Can you work these out from the model? Positions are in its coordinate system, mm. A direction names the side the tool comes from. Give positions to 0.01 mm unless a question says otherwise; leave off trailing zeros. Loops run counter-clockwise (first coordinate to the right, second up) from the corner with the lowest first, then second, coordinate; pieces in that order, holes last. Notation, with made-up numbers: (14.5, -32.75) -> (57.5, -32.75) arc R19 cw to (57.5, -22.75) -> close; hole circle Ø4 at (72, 81.5). An arc over 180 degrees is marked (long way). Use CSV: the item, a comma, the result in double quotes.
from build123d import *

# Parameters (mm, degrees)
SKIZZE1_W                            = 100
SKIZZE1_H                            = 25
AUFSATZ_LINEAR_AUSTRAGEN1_DEPTH      = 3
SKIZZE3_W                            = 4
SKIZZE3_H                            = 17
AUFSATZ_LINEAR_AUSTRAGEN2_DEPTH      = 17
SCHNITT_LINEAR_AUSTRAGEN1_DEPTH      = 78.95222289
SCHNITT_LINEAR_AUSTRAGEN1_DEPTH_BACK = 78.95222289
SKIZZE5_R                            = 2.55
VERRUNDUNG1_R                        = 8.5
SKIZZE6_R                            = 2.6
SCHNITT_LINEAR_AUSTRAGEN2_DEPTH      = 3
VERRUNDUNG2_R                        = 1


with BuildPart() as part:
    # Skizze1 → Aufsatz-Linear austragen1 (new body)
    with BuildSketch(Plane.XY):
        with Locations((45.947748482, 6.142667555)):
            Rectangle(SKIZZE1_W, SKIZZE1_H)
    extrude(amount=AUFSATZ_LINEAR_AUSTRAGEN1_DEPTH)

    # Skizze3 → Aufsatz-Linear austragen2 (add)
    with BuildSketch(Plane.XY.offset(3)):
        with Locations((12.947748482, 6.142667555)):
            Rectangle(SKIZZE3_W, SKIZZE3_H)
        with Locations((20.947748482, 6.142667555)):
            Rectangle(SKIZZE3_W, SKIZZE3_H)
        with Locations((78.947748482, 6.142667555)):
            Rectangle(SKIZZE3_W, SKIZZE3_H)
        with Locations((70.947748482, 6.142667555)):
            Rectangle(SKIZZE3_W, SKIZZE3_H)
    extrude(amount=AUFSATZ_LINEAR_AUSTRAGEN2_DEPTH)

    # Skizze5 → Schnitt-Linear austragen1 (cut, two sides: drawn at the far end of the back side and taken through both)
    with BuildSketch(Plane(origin=(22.947748482, 0, 0), x_dir=(0, 0, -1), z_dir=(1, 0, 0)).offset(-SCHNITT_LINEAR_AUSTRAGEN1_DEPTH_BACK)):
        with Locations(Location((-11.5, 6.142667555, 0), (0, 0, 90))):
            Circle(SKIZZE5_R)
    extrude(amount=SCHNITT_LINEAR_AUSTRAGEN1_DEPTH + SCHNITT_LINEAR_AUSTRAGEN1_DEPTH_BACK, mode=Mode.SUBTRACT)

    # Verrundung1
    verrundung1_edges = [part.edges().sort_by_distance(p)[0] for p in [
        (20.947748482, 14.642667555, 20),
        (12.947748482, 14.642667555, 20),
        (12.947748482, -2.357332445, 20),
        (20.947748482, -2.357332445, 20),
        (78.947748482, 14.642667555, 20),
        (70.947748482, 14.642667555, 20),
        (70.947748482, -2.357332445, 20),
        (78.947748482, -2.357332445, 20),
    ]]
    fillet(verrundung1_edges, radius=VERRUNDUNG1_R - 0.0001)  # a hair under: the kernel refuses the full size

    # Skizze6 → Schnitt-Linear austragen2 (cut)
    with BuildSketch(Plane.XY.offset(3)):
        with Locations((2.947748482, 6.142667555)):
            Circle(SKIZZE6_R)
        with Locations(Location((88.947748482, 6.142667555, 0), (0, 0, 180))):
            Circle(SKIZZE6_R)
    extrude(amount=-SCHNITT_LINEAR_AUSTRAGEN2_DEPTH, mode=Mode.SUBTRACT)

    # Verrundung2
    verrundung2_edges = [part.edges().sort_by_distance(p)[0] for p in [
        (95.947748482, -6.357332445, 1.5),
        (95.947748482, 18.642667555, 1.5),
        (-4.052251518, 18.642667555, 1.5),
        (-4.052251518, -6.357332445, 1.5),
    ]]
    fillet(verrundung2_edges, radius=VERRUNDUNG2_R)


solid = part.part
(1) Will these pins go through, and if not, where does the flat tip stop? pin 1 Ø5 at (y, z) = (2, 12.5) entering from +X; pin 2 Ø3 at (y, z) = (7, 10.5) entering from -X; pin 3 Ø6 at (x, z) = (22.5, 10.5) entering from -Y; pin 4 Ø10 at (x, z) = (20.5, 5.5) entering from -Y.
Answer sheet:
pin 1,"stops at x = 80.95"
pin 2,"stops at x = 10.95"
pin 3,"stops at y = -2.36"
pin 4,"stops at y = -6.36"
(2) If we section it at B-B, the plane y = 0: Write out the boundary of the cut face in (x, z).
Answer sheet:
outline,"(-4.05, 0) -> (95.95, 0) -> (95.95, 3) -> (80.95, 3) -> (80.95, 17.38) -> (76.95, 17.38) -> (76.95, 3) -> (72.95, 3) -> (72.95, 17.38) -> (68.95, 17.38) -> (68.95, 3) -> (22.95, 3) -> (22.95, 17.38) -> (18.95, 17.38) -> (18.95, 3) -> (14.95, 3) -> (14.95, 17.38) -> (10.95, 17.38) -> (10.95, 3) -> (-4.05, 3) -> close"
(3) If I drill on L1, parallel to X at y = 14.25, z = 11.75; L2, parallel to Y at x = 14.5, z = 11.75; L3, parallel to X at y = 5.25, z = 2.25, over which ranges is the centre line in solid material (lowest first)? Write a range as from..to.
Answer sheet:
L1,"x = 10.95..14.95, 18.95..22.95, 68.95..72.95, 76.95..80.95"
L2,"y = -2.35..3.6, 8.68..14.64"
L3,"x = -4.05..0.51, 5.39..86.51, 91.39..95.95"
(4) If we section it at D-D, the plane y = 16.25: Write out the boundary of the cut face in (x, z), then the cut area to 3 significant figures.
Answer sheet:
outline,"(-4.05, 0) -> (95.95, 0) -> (95.95, 3) -> (-4.05, 3) -> close"
area,"300 mm2"
(5) We'd pull the mould along X, two halves only. Please class faces 4 (the face through (20.976, 0.067, 17.444)), 5 (the face through (95.948, 6, 1)), 6 (the face through (22.948, 8, 9)): released by +X, released by -X, zero draft, split by the parting line, or undercut.
Answer sheet:
face 4,"zero draft"
face 5,"released by +X"
face 6,"undercut"
(6) If we section it at A-A, the plane z = 12.75: Give the number of separate pieces and of enclosed holes in the cut face, then the cut area to 3 significant figures.
Answer sheet:
separate pieces,"8"
enclosed holes,"0"
area,"198 mm2"
(7) Which directions (+Z, -Z, +X, -X, +Y, -Y) give clear straight access to the entire face, cutting with the end or side of a thin tool? Please do faces 1 (the face through (13, 14.643, 7)), 2 (the face through (14.948, 8, 9)), 3 (the face through (80.948, 8, 9)).
Answer sheet:
face 1,"+Z, +X, -X, +Y"
face 2,"+Z, +Y, -Y"
face 3,"+Z, +X, +Y, -Y"
(8) If we section it at C-C, the plane x = 51: Write out the boundary of the cut face in (y, z).
Answer sheet:
outline,"(-6.36, 0) -> (18.64, 0) -> (18.64, 3) -> (-6.36, 3) -> close"
